Build history of the part. All positions in model axes, mm. A direction names the side the tool comes from. Coordinates: 2 decimals unless noted, no trailing zeros. Write each loop counter-clockwise with the first axis right and the second up, starting at its lowest first coordinate (ties: lowest second). Pieces come first, ordered by that corner, then holes.
from build123d import *

# Parameters (mm, degrees)
F1_DEPTH = 10
F3_DEPTH = 170
F4_W     = 4.053228
F4_H     = 4.812476
F5_DEPTH = 25
F6_W     = 4.812476
F6_H     = 10
F7_DEPTH = 1.55
F8_R     = 8.5
F9_DEPTH = 1


with BuildPart() as f1:
    # F0 (on Top) → F1 (new body)
    with BuildSketch(Plane.XY):
        with BuildLine():
            Line((0, -66.863723), (13.439171, -66.863723))
            ThreePointArc((13.439171, -66.863723), (68.190366, 1.201156), (11.07599, 67.295551))
            Line((11.07599, 67.295551), (0, 67.295551))
            Line((0, 67.295551), (-11.07599, 67.295551))
            ThreePointArc((-11.07599, 67.295551), (-68.190366, 1.201156), (-13.439171, -66.863723))
            Line((-13.439171, -66.863723), (0, -66.863723))
        make_face()
        with BuildLine():
            Line((-11.445523, 65), (0, 65))
            Line((0, 65), (11.445523, 65))
            ThreePointArc((11.445523, 65), (50.553954, 42.429916), (66, 0))
            ThreePointArc((66, 0), (50.553954, -42.429916), (11.445523, -65))
            Line((11.445523, -65), (0, -65))
            Line((0, -65), (-11.445523, -65))
            ThreePointArc((-11.445523, -65), (-50.553954, -42.429916), (-66, 0))
            ThreePointArc((-66, 0), (-50.553954, 42.429916), (-11.445523, 65))
        make_face(mode=Mode.SUBTRACT)
    extrude(amount=F1_DEPTH)

    # F2 (on face) → F3 (cut)
    with BuildSketch(Plane(origin=(0, 67.295551, 0), x_dir=(-1, 0, 0), z_dir=(0, 1, 0))):
        with BuildLine():
            ThreePointArc((0, 6.875), (-1.875, 5), (0, 3.125))
            Line((0, 3.125), (0, 6.875))
        make_face()
        with BuildLine():
            Line((0, 6.875), (0, 3.125))
            ThreePointArc((0, 3.125), (1.325825, 3.674175), (1.875, 5))
            ThreePointArc((1.875, 5), (1.325825, 6.325825), (0, 6.875))
        make_face()
    extrude(amount=-F3_DEPTH, mode=Mode.SUBTRACT)

    # F4 (on face) → F5 (cut)
    with BuildSketch(Plane.XY.offset(10)):
        with Locations((-68.636846, 0)):
            Rectangle(F4_W, F4_H)
    extrude(amount=-F5_DEPTH, mode=Mode.SUBTRACT)

    # F6 (on face) → F7 (join)
    with BuildSketch(Plane(origin=(-66.610232, 0, 0), x_dir=(0, -1, 0), z_dir=(-1, 0, 0))):
        with Locations((0, 5)):
            Rectangle(F6_W, F6_H)
    extrude(amount=F7_DEPTH)

    # F8 (on face) → F9 (cut)
    with BuildSketch(Plane(origin=(-68.160232, 0, 0), x_dir=(0, -1, 0), z_dir=(-1, 0, 0))):
        with Locations((0, 5)):
            Circle(F8_R)
    extrude(amount=-F9_DEPTH, mode=Mode.SUBTRACT)


solid = f1.part
(1) Flat gauge pins, fed straight in: P1, Ø1, axis at y = 2, z = 7, coming from the -X side; P2, Ø5, axis at y = -50.5, z = 8.5, coming from the +X side. Where does each tip first touch, or does it go through?
(2) Slice it at B-B, the plane y = -26. List the corners of the cut face in (x, z), and give its area (3 significant figures).
(3) Slice it at A-A, the plane x = -7. List the corners of the cut face in (y, z).
(4) Probe L1, parallel to Y at x = 3.5, z = 1.25; L2, parallel to X at y = 23, z = 6.75; L3, parallel to Y at x = -30, z = 8.25. List the from-to ranges inside material, lowest first.
(5) 3-axis set-ups, long thin cutter, end or side, ignore diameter. For faces 4 (the flat face through (-67.16, 0, 5)), 5 (the flat face through (0.2, -65, 2.7)), 6 (the flat face through (-0.2, -66.864, 2.7)): which of +Z, -Z, +X, -X, +Y, -Y reach the whole face in a straight line?
(6) Two-plate mould, pull along X, no slides. Class faces 1 (the cylindrical face through (-50.92, -45.37, 4.93)), 2 (the cylindrical face through (68.2, -0.1, 4.9)), 3 (the flat face through (-0.2, 65, 2.7)): pulls with the +X half, pulls with the -X half, needs draft (parallel to the pull), parting line crosses it, or undercut.
Results:
1. P1: stops at x = -67.16
1. P2: stops at x = 48.45
2. outline: (-63.05, 0) - (-60.66, 0) - (-60.66, 10) - (-63.05, 10) - close; (60.66, 0) - (63.05, 0) - (63.05, 10) - (60.66, 10) - close
2. area: 47.8 mm2
3. outline: (-66.86, 0) - (-65, 0) - (-65, 10) - (-66.86, 10) - close; (65, 0) - (67.3, 0) - (67.3, 10) - (65, 10) - close
4. L1: y = -66.86 to -65, 65 to 67.3
4. L2: x = -64.21 to -61.86, 61.86 to 64.21
4. L3: y = -61.25 to -58.79, 58.79 to 61.25
5. face 4: -X
5. face 5: +Z, -Z
5. face 6: +Z, -Z, +X, -X, -Y
6. face 1: pulls with the -X half
6. face 2: pulls with the +X half
6. face 3: undercut
